Design review of the part built by this model. Coordinates are the model's own, in mm. Round coordinates to 2 decimals unless told otherwise and drop trailing zeros. Loops run counter-clockwise (first coordinate to the right, second up) from the corner with the lowest first, then second, coordinate; pieces in that order, holes last. Notation, with made-up numbers: (-27, -32.5) - (-2, -32.5) arc R22 ccw to (-2, -4.5) - close; hole circle Ø6 at (-18, 64.25). An arc over 180 degrees is marked (long way). One line per question, with ' | ' between items. Start each with the question number.
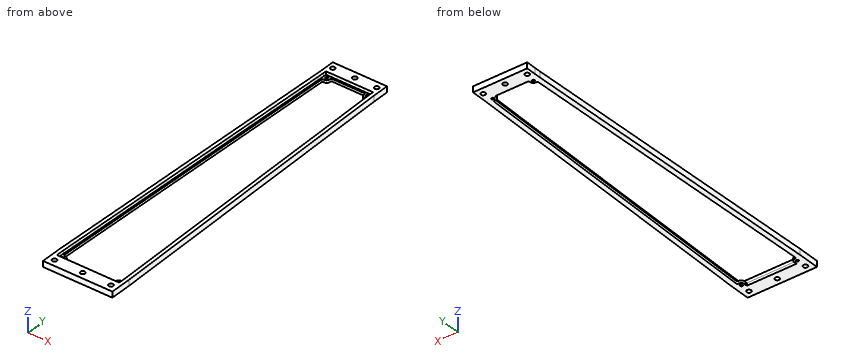
from build123d import *

# Parameters (mm, degrees)
SKETCH_2_R      = 1
EXTRUDE_1_DEPTH = 2
EXTRUDE_2_DEPTH = 2
EXTRUDE_3_DEPTH = 2.5
SKETCH_5_R      = 1.75
EXTRUDE_4_DEPTH = 4.5


with BuildPart() as part:
    # 草图2 → 凸台-拉伸1 (new body)
    with BuildSketch(Plane(origin=(0, 0, -1.538354077), x_dir=(-1, 0, 0), z_dir=(0, 0, -1))):
        with BuildLine():
            Line((-22.942959106, -124.662212149), (-17.134907671, 121.132350923))
            ThreePointArc((-17.134907671, 121.132350923), (-16.793190136, 121.861742775), (-16.024570953, 122.102591063))
            ThreePointArc((-16.024570953, 122.102591063), (-14.009380987, 122.790837638), (-13.255665128, 124.782466708))
            ThreePointArc((-13.255665128, 124.782466708), (-12.992914403, 125.539491489), (-12.25871858, 125.860553721))
            Line((-12.25871858, 125.860553721), (12.25871858, 125.860553721))
            ThreePointArc((12.25871858, 125.860553721), (12.992914403, 125.539491489), (13.255665128, 124.782466708))
            ThreePointArc((13.255665128, 124.782466708), (14.009380087, 122.79083851), (16.024568463, 122.102590786))
            ThreePointArc((16.024568463, 122.102590786), (16.793187022, 121.861742062), (17.134904184, 121.13235055))
            Line((17.134904184, 121.13235055), (22.942959106, -124.662212156))
            Line((22.942959106, -124.662212156), (22.942959106, -124.904555532))
            ThreePointArc((22.942959106, -124.904555532), (22.626864313, -125.634126411), (21.878411771, -125.902470178))
            ThreePointArc((21.878411771, -125.902470178), (19.586380534, -127.089481736), (19.565603095, -129.670561341))
            Line((19.565603095, -129.670561341), (19.265011022, -129.670561341))
            Line((19.265011022, -129.670561341), (19.265011022, -130.670561341))
            Line((19.265011022, -130.670561341), (23.942959106, -130.670561341))
            Line((23.942959106, -130.670561341), (23.942959106, -124.650398948))
            Line((23.942959106, -124.650398948), (18.052063488, 124.649948906))
            Line((18.052063488, 124.649948906), (18.052059944, 126.860553721))
            Line((18.052059944, 126.860553721), (-18.052059944, 126.860553721))
            Line((-18.052059944, 126.860553721), (-18.052059944, 124.65024892))
            Line((-18.052059944, 124.65024892), (-23.942959106, -124.650398948))
            Line((-23.942959106, -124.650398948), (-23.942959106, -130.670561341))
            Line((-23.942959106, -130.670561341), (-19.234988978, -130.670561341))
            Line((-19.234988978, -130.670561341), (-19.234988978, -129.670561341))
            Line((-19.234988978, -129.670561341), (-19.646017972, -129.670561341))
            ThreePointArc((-19.646017972, -129.670561341), (-19.548027097, -127.027128176), (-21.878411771, -125.775469924))
            ThreePointArc((-21.878411771, -125.775469924), (-22.626864313, -125.507126157), (-22.942959106, -124.777555278))
            Line((-22.942959106, -124.777555278), (-22.942959106, -124.662212149))
        make_face()
        with Locations((-21.717043434, -128.270256541)):
            Circle(SKETCH_2_R, mode=Mode.SUBTRACT)
        with Locations((21.717043434, -128.397256794)):
            Circle(SKETCH_2_R, mode=Mode.SUBTRACT)
        with Locations((-15.748031496, 124.587249174)):
            Circle(SKETCH_2_R, mode=Mode.SUBTRACT)
        with Locations((15.748031496, 124.587249174)):
            Circle(SKETCH_2_R, mode=Mode.SUBTRACT)
    extrude(amount=EXTRUDE_1_DEPTH)

    # 草图3 → 凸台-拉伸2 (add)
    with BuildSketch(Plane(origin=(0, 0, -3.538354077), x_dir=(-1, 0, 0), z_dir=(0, 0, -1))):
        Polygon((26.942959106, -124.614959326), (21.052063431, 124.685390934), (21.052055134, 129.860553721), (-21.052059944, 129.860553721), (-21.052059944, 124.685688522), (-26.942959106, -124.614959347), (-26.942959106, -133.670561341), (26.942959106, -133.670561341), align=None)
        Polygon((18.052059944, 126.860553721), (-18.052059944, 126.860553721), (-18.052059944, 124.65024892), (-23.942959106, -124.650398948), (-23.942959106, -130.670561341), (23.942959106, -130.670561341), (23.942959106, -124.650398948), (18.052063488, 124.649948906), align=None, mode=Mode.SUBTRACT)
    extrude(amount=-EXTRUDE_2_DEPTH)

    # 草图4 → 凸台-拉伸3 (add)
    with BuildSketch(Plane.XY.offset(-1.538354077)):
        Polygon((-21.052063431, 124.685390934), (-26.942959106, -124.614959326), (-26.942959106, -133.670561341), (26.942959106, -133.670561341), (26.942959106, -124.614959347), (21.052059944, 124.685688522), (21.052059944, 129.860553721), (-21.052055134, 129.860553721), align=None)
        Polygon((-18.302059543, 127.110553721), (-18.302063484, 124.652902409), (-24.192959106, -124.647445647), (-24.192959106, -130.920561341), (24.192959106, -130.920561341), (24.192959106, -124.647445648), (18.302059944, 124.653202221), (18.302059944, 127.110553721), align=None, mode=Mode.SUBTRACT)
    extrude(amount=EXTRUDE_3_DEPTH)

    # 草图5 → 凸台-拉伸4 (add)
    # profile 1 of 2: a face of its own
    with BuildSketch(Plane.XY.offset(0.961645923)):
        Polygon((-26.942959106, -133.670561341), (26.942959106, -133.670561341), (26.942959106, -138.670561341), (26.942959106, -141.170561341), (-26.942959106, -141.170561341), (-26.942959106, -138.670561341), align=None)
        with Locations((2.405e-06, -136.170561341)):
            Circle(SKETCH_5_R, mode=Mode.SUBTRACT)
        with Locations((21.942959106, -136.170561341)):
            Circle(SKETCH_5_R, mode=Mode.SUBTRACT)
        with Locations((-21.942959106, -136.170561341)):
            Circle(SKETCH_5_R, mode=Mode.SUBTRACT)
    # profile 2 of 2: a face of its own
    with BuildSketch(Plane.XY.offset(0.961645923)):
        Polygon((21.052059944, 129.860553721), (-21.052055134, 129.860553721), (-21.052055134, 134.860553721), (-21.052055134, 137.360553721), (21.052059944, 137.360553721), (21.052059944, 134.860553721), align=None)
        with Locations((-17.052055134, 132.360553721)):
            Circle(SKETCH_5_R, mode=Mode.SUBTRACT)
        with Locations((17.052059944, 132.360553721)):
            Circle(SKETCH_5_R, mode=Mode.SUBTRACT)
        with Locations((2.405e-06, 132.360553721)):
            Circle(SKETCH_5_R, mode=Mode.SUBTRACT)
    extrude(amount=-EXTRUDE_4_DEPTH)


solid = part.part
1. Clearance check with flat-ended pins moving along their axes: P1, Ø2.5, axis at y = 126, z = -0.5, coming from the -X side; P2, Ø2, axis at y = 55.5, z = -3, coming from the -X side; P3, Ø2, axis at y = 126.5, z = -1, coming from the +X side. State where each tip first meets the part, or that it passes through.
2. To check wall thickness, follow line 1 along Y through (x, z) = (17, 0.2); line 2 along Y through (x, z) = (13, -1.85); line 3 along Y through (x, z) = (-16, -0.5). State the ranges of each line that lie inside material, in increasing order.
3. Take a section at C-C, the plane z = 0.1. Give the boundary of the cut face in (x, y), then the cut area to 3 significant figures.
4. Take a section at A-A, the plane x = -8. Give the boundary of the cut face in (y, z), then the cut area to 4 significant figures.
5. Take a section at B-B, the plane y = -87. Give the boundary of the cut face in (x, z), then the cut area to 3 significant figures.
Answer list:
1) P1: stops at x = -21.05 | P2: stops at x = -22.71 | P3: stops at x = 21.05
2) line 1: y = -141.17 to -130.92, 127.11 to 130.61, 134.11 to 137.36 | line 2: y = -141.17 to -130.67, 125.53 to 137.36 | line 3: y = -141.17 to -130.92, 127.11 to 130.96, 133.76 to 137.36
3) outline: (-26.94, -141.17) - (26.94, -141.17) - (26.94, -124.61) - (21.05, 124.69) - (21.05, 137.36) - (-21.05, 137.36) - (-21.05, 129.86) - (-21.05, 124.69) - (-26.94, -124.61) - close; hole (-24.19, -130.92) - (24.19, -130.92) - (24.19, -124.65) - (18.3, 124.65) - (18.3, 127.11) - (-18.3, 127.11) - (-18.3, 124.65) - (-24.19, -124.65) - close; hole circle Ø3.5 at (-21.94, -136.17); hole circle Ø3.5 at (-17.05, 132.36); hole circle Ø3.5 at (0, -136.17); hole circle Ø3.5 at (0, 132.36); hole circle Ø3.5 at (17.05, 132.36); hole circle Ø3.5 at (21.94, -136.17) | area: 2,350 mm²
4) outline: (-141.17, -3.54) - (-130.67, -3.54) - (-130.67, -1.54) - (-130.92, -1.54) - (-130.92, 0.96) - (-141.17, 0.96) - close; (125.86, -3.54) - (137.36, -3.54) - (137.36, 0.96) - (127.11, 0.96) - (127.11, -1.54) - (125.86, -1.54) - close | area: 95.25 mm²
5) outline: (-26.05, -3.54) - (-22.05, -3.54) - (-22.05, -1.54) - (-23.3, -1.54) - (-23.3, 0.96) - (-26.05, 0.96) - close; (22.05, -3.54) - (26.05, -3.54) - (26.05, 0.96) - (23.3, 0.96) - (23.3, -1.54) - (22.05, -1.54) - close | area: 29.8 mm²
